Part model, mm, in its own coordinate system. A direction names the side the tool comes from. Round coordinates to 2 decimals unless told otherwise and drop trailing zeros. Order: outer loops, then holes, each group sorted by start corner. A loop starts at its lowest first (then second) coordinate and runs counter-clockwise, first axis right, second up. Notation, with made-up numbers: M -0.75,11.25 L 36.25,11.25 A32 ccw 36.25,43.25 Z; hole C -25.75,12.25 d3. An arc over 180 degrees is marked long. One line per question, with ' | ' between items.
Autodesk Inventor part; units mm, degrees
ref_plane "YZ Plane" through (0, 0, 0) normal (1, 0, 0) x (0, 1, 0)
ref_plane "XZ Plane" through (0, 0, 0) normal (0, 1, 0) x (-1, 0, 0)
ref_plane "XY Plane" through (0, 0, 0) normal (0, 0, 1) x (1, 0, 0)
sketch "Sketch1" plane through (0, 0, 0) normal (0, 1, 0) x (-1, 0, 0)
  line L0 (-5, 25) -> (-5, -25)
  line L1 (-5, -25) -> (5, -25)
  line L2 (5, -25) -> (5, 25)
  line L3 (5, 25) -> (-5, 25)
  line L4 (-5, 25) -> (5, -25) construction
  line L5 (-5, -25) -> (5, 25) construction
  point P0 (0, 0)
  dimension "d0" = 50
  dimension "d1" = 10
extrude "Extrusion1" add sketch "Sketch1" along normal blind 0.5
sketch "Sketch2" plane through (0, 0.5, 0) normal (0, 1, 0) x (1, 0, 0)
  line L0 (2.5, -2.5) -> (2.5, 2.5)
  line L1 (2.5, 2.5) -> (-2.5, 2.5)
  line L2 (-2.5, 2.5) -> (-2.5, -2.5)
  line L3 (-2.5, -2.5) -> (2.5, -2.5)
  line L4 (2.5, -2.5) -> (-2.5, 2.5) construction
  line L5 (2.5, 2.5) -> (-2.5, -2.5) construction
  line L6 (-5, -25) -> (5, -25)
  line L7 (0, -25) -> (0, -17)
  line L8 (2.5, -19.5) -> (2.5, -14.5)
  line L9 (2.5, -14.5) -> (-2.5, -14.5)
  line L10 (-2.5, -14.5) -> (-2.5, -19.5)
  line L11 (-2.5, -19.5) -> (2.5, -19.5)
  line L12 (2.5, -19.5) -> (-2.5, -14.5) construction
  line L13 (2.5, -14.5) -> (-2.5, -19.5) construction
  line L14 (5, 25) -> (-5, 25)
  line L15 (0, 25) -> (0, 17)
  line L16 (2.5, 14.5) -> (2.5, 19.5)
  line L17 (2.5, 19.5) -> (-2.5, 19.5)
  line L18 (-2.5, 19.5) -> (-2.5, 14.5)
  line L19 (-2.5, 14.5) -> (2.5, 14.5)
  line L20 (2.5, 14.5) -> (-2.5, 19.5) construction
  line L21 (2.5, 19.5) -> (-2.5, 14.5) construction
  point P0 (0, 0)
  dimension "d4" = 5
  dimension "d5" = 5
  dimension "d6" = 8
  dimension "d7" = 5
  dimension "d8" = 5
  dimension "d9" = 8
  dimension "d10" = 5
extrude "Extrusion2" add sketch "Sketch2" along normal blind 1
sketch "Sketch3" plane through (0, 0.5, 0) normal (0, 1, 0) x (1, 0, 0)
  line L0 (-5, -25) -> (5, -25)
  line L1 (0, -25) -> (0, -11)
  line L2 (1.7, -11.65) -> (1.7, -10.35)
  line L3 (1.7, -10.35) -> (-1.7, -10.35)
  line L4 (-1.7, -10.35) -> (-1.7, -11.65)
  line L5 (-1.7, -11.65) -> (1.7, -11.65)
  line L6 (1.7, -11.65) -> (-1.7, -10.35) construction
  line L7 (1.7, -10.35) -> (-1.7, -11.65) construction
  line L8 (0, -11) -> (0, -6)
  line L9 (1.9118, -6.65) -> (-1.9118, -6.65)
  line L10 (-1.9118, -6.65) -> (-1.9118, -5.35)
  line L11 (-1.9118, -5.35) -> (1.9118, -5.35)
  line L12 (1.9118, -5.35) -> (1.9118, -6.65)
  line L13 (1.9118, -6.65) -> (-1.9118, -5.35) construction
  line L14 (-1.9118, -6.65) -> (1.9118, -5.35) construction
  line L15 (2.5, 2.5) -> (-2.5, 2.5)
  line L16 (0, 2.5) -> (0, 8.5)
  line L17 (1.9118, 7.85) -> (-1.9118, 7.85)
  line L18 (-1.9118, 7.85) -> (-1.9118, 9.15)
  line L19 (-1.9118, 9.15) -> (1.9118, 9.15)
  line L20 (1.9118, 9.15) -> (1.9118, 7.85)
  line L21 (1.9118, 7.85) -> (-1.9118, 9.15) construction
  line L22 (-1.9118, 7.85) -> (1.9118, 9.15) construction
  point P0 (0, 0)
  dimension "d13" = 14
  dimension "d14" = 1.3
  dimension "d15" = 3.4
  dimension "d16" = 5
  dimension "d17" = 1.3
  dimension "d18" = 6
  dimension "d19" = 1.3
extrude "Extrusion3" add sketch "Sketch3" along normal blind 0.5
sketch "Sketch4" plane through (0, 1.5, 0) normal (0, 1, 0) x (1, 0, 0)
  circle A0 centre (0, 0) radius 2
  circle A1 centre (0, -17) radius 2
  circle A2 centre (0, 17) radius 2
  dimension "d22" = 4
  dimension "d23" = 4
  dimension "d24" = 4
extrude "Extrusion4" cut sketch "Sketch4" against normal blind 0.1
properties part number "5050-led-strip"
1) Two-plate mould, pull along Z, no slides. Class faces 1 (the face through (-2.5, 1, -17)), 2 (the face through (0, 1, 19.5)), 3 (the face through (0, 1, -14.5)): released by +Z, released by -Z, zero draft, split by the parting line, or undercut.
The answers:
face 1: zero draft | face 2: released by +Z | face 3: undercut
2) Drop flat-ended pins along their axis: pin 1 (5 mm diameter, centred on x = -2.5, z = -9.5, fed in from +Y); pin 2 (0.5 mm diameter, centred on x = -1, y = 1, fed in from +Z); pin 3 (0.5 mm diameter, centred on y = 1, z = -1, fed in from +X). Give the stop position or say it passes through.
The answers:
pin 1: stops at y = 1 | pin 2: stops at z = 19.5 | pin 3: stops at x = 2.5
3) Saw through at A-A (y = 0.75). List the corners of the cut face in (x, z), plus the area to 3 significant figures.
The answers:
outline: M -2.5,-19.5 L 2.5,-19.5 L 2.5,-14.5 L -2.5,-14.5 Z; M -2.5,-2.5 L 2.5,-2.5 L 2.5,2.5 L -2.5,2.5 Z; M -2.5,14.5 L 2.5,14.5 L 2.5,19.5 L -2.5,19.5 Z; M -1.91,-9.15 L 1.91,-9.15 L 1.91,-7.85 L -1.91,-7.85 Z; M -1.91,5.35 L 1.91,5.35 L 1.91,6.65 L -1.91,6.65 Z; M -1.7,10.35 L 1.7,10.35 L 1.7,11.65 L -1.7,11.65 Z | area: 89.4 mm²
4) Saw through at D-D (z = 1). List the corners of the cut face in (x, y).
The answers:
outline: M -5,0 L 5,0 L 5,0.5 L 2.5,0.5 L 2.5,1.5 L 1.73,1.5 L 1.73,1.4 L -1.73,1.4 L -1.73,1.5 L -2.5,1.5 L -2.5,0.5 L -5,0.5 Z
5) Saw through at B-B (z = -17). List the corners of the cut face in (x, y).
The answers:
outline: M -5,0 L 5,0 L 5,0.5 L 2.5,0.5 L 2.5,1.5 L 2,1.5 L 2,1.4 L -2,1.4 L -2,1.5 L -2.5,1.5 L -2.5,0.5 L -5,0.5 Z
6) Probe line 1 (Z direction, x = 0.75, y = 0.85); line 2 (Z direction, x = -1.25, y = 1.35); line 3 (Y direction, x = -4, z = -13.5). List the from-to ranges inside material, lowest first. Write a range as [from, to].
The answers:
line 1: z = [-19.5, -14.5], [-9.15, -7.85], [-2.5, 2.5], [5.35, 6.65], [10.35, 11.65], [14.5, 19.5] | line 2: z = [-19.5, -14.5], [-2.5, 2.5], [14.5, 19.5] | line 3: y = [0, 0.5]
7) Saw through at C-C (x = 4). List the corners of the cut face in (y, z), plus the area to 3 significant figures.
The answers:
outline: M 0,-25 L 0.5,-25 L 0.5,25 L 0,25 Z | area: 25.0 mm²
8) Which spindle directions (+Z, -Z, +X, -X, +Y, -Y) get a long thin tool onto all of the face, cutting with end or side? Do faces 4 (the face through (0, 1, -9)), 5 (the face through (-2.5, 1, 0)), 6 (the face through (0, 1.4, -17)), 7 (the face through (2.5, 1, 17)). Say none if no direction does.
The answers:
face 4: +X, -X, +Y | face 5: +Z, -Z, -X, +Y | face 6: +Y | face 7: +Z, -Z, +X, +Y
